The figure shows three views and two pictorial views of one solid part (mm, origin at its lowest corner). Answer the questions. A direction names the side the tool comes from. Give positions to 0.01 mm unless a question says otherwise; leave off trailing zeros. Write each loop counter-clockwise with the first axis right and the second up, starting at its lowest first coordinate (ties: lowest second). Pieces come first, ordered by that corner, then holes. Notation, with made-up numbers: M 17,69 L 45,69 A14 ccw 45,85 Z; hole C 5,81 d6. An arc over 180 degrees is marked long. Return JSON: item names as keys, results as strings.
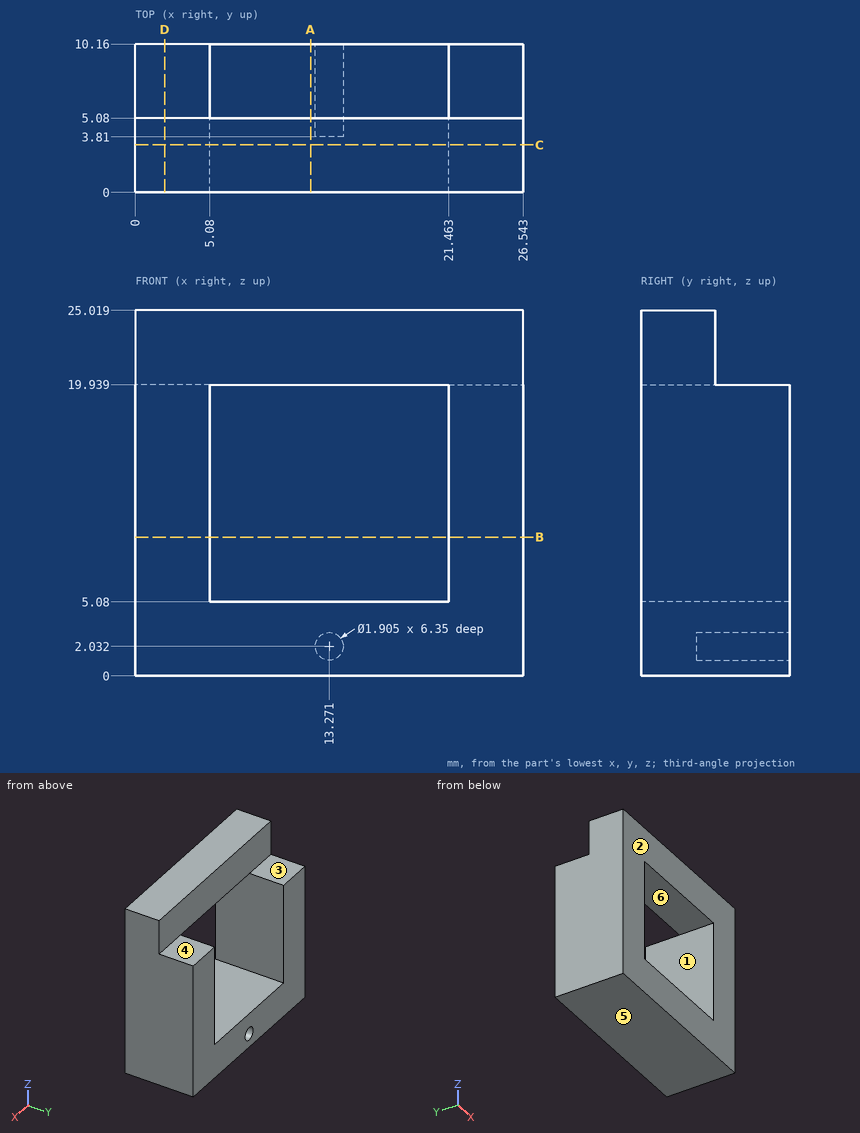
Item 1: A cutting plane is placed at B-B, the plane z = 9.5. Write down the section's boundary in (x, y), plus the area to 3 significant figures.
Geometry results:
{"outline": "M 0,0 L 5.08,0 L 5.08,10.16 L 0,10.16 Z; M 21.46,0 L 26.54,0 L 26.54,10.16 L 21.46,10.16 Z", "area": "103 mm2"}
Item 2: Given pin 1 Ø1.5 at (x, z) = (13.27, 2.03) entering from +Y; pin 2 Ø1.5 at (x, z) = (9.5, 23) entering from +Y; pin 3 Ø5.5 at (x, y) = (2.5, 9) entering from +Z, each flat-ended and moving along its own axis, determine where each tip first touches the part or whether it passes through.
Geometry results:
{"pin 1": "stops at y = 3.81", "pin 2": "stops at y = 5.08", "pin 3": "stops at z = 19.94"}
Item 3: Which of the six approach directions +Z, -Z, +X, -X, +Y, -Y give full straight-line access (tool end or side, diameter ignored) to the marked faces 4, 5 and 6?
Geometry results:
{"face 4": "+Z, +X, -X, +Y", "face 5": "-Z, +X, -X, +Y, -Y", "face 6": "+Y, -Y"}
Item 4: A cutting plane is placed at D-D, the plane x = 2. Write down the section's boundary in (y, z), plus the area to 3 significant figures.
Geometry results:
{"outline": "M 0,0 L 10.16,0 L 10.16,19.94 L 5.08,19.94 L 5.08,25.02 L 0,25.02 Z", "area": "228 mm2"}
Item 5: Find the intervals of material crossed by line 1 (X direction, y = 2.5, z = 7.5); line 2 (Z direction, x = 15, y = 1); line 3 (Z direction, x = 6.75, y = 6.25), in increasing order.
Geometry results:
{"line 1": "x = 0 to 5.08, 21.46 to 26.54", "line 2": "z = 0 to 5.08, 19.94 to 25.02", "line 3": "z = 0 to 5.08"}
Item 6: Determine the mould class of the marked faces 1, 2 and 3 for opening direction Z: +Z half, -Z half, draft (parallel to the pull), parting line (faces both ways), or undercut.
Geometry results:
{"face 1": "undercut", "face 2": "draft", "face 3": "+Z half"}
Item 7: A cutting plane is placed at A-A, the plane x = 12. Write down the section's boundary in (y, z).
Geometry results:
{"outline": "M 0,0 L 10.16,0 L 10.16,5.08 L 0,5.08 Z; M 0,19.94 L 5.08,19.94 L 5.08,25.02 L 0,25.02 Z"}
Item 8: A cutting plane is placed at C-C, the plane y = 3.25. Write down the section's boundary in (x, z).
Geometry results:
{"outline": "M 0,0 L 26.54,0 L 26.54,25.02 L 0,25.02 Z; hole M 5.08,5.08 L 21.46,5.08 L 21.46,19.94 L 5.08,19.94 Z"}
